Autodesk Inventor part; units mm, degrees
ref_plane "YZ Plane" through (0, 0, 0) normal (1, 0, 0) x (0, 1, 0)
ref_plane "XZ Plane" through (0, 0, 0) normal (0, 1, 0) x (-1, 0, 0)
ref_plane "XY Plane" through (0, 0, 0) normal (0, 0, 1) x (1, 0, 0)
sketch "Esquisse1" plane through (0, 0, 0) normal (0, 1, 0) x (-1, 0, 0)
  line L0 (0, 0) -> (37, 0)
  line L1 (37, 0) -> (37, -31.5)
  line L2 (37, -31.5) -> (0, -31.5)
  line L3 (0, -31.5) -> (0, 0)
  line L4 (34, -28.5) -> (34, -3)
  line L5 (34, -3) -> (3, -3)
  line L6 (3, -3) -> (3, -28.5)
  line L7 (3, -28.5) -> (34, -28.5)
  line L8 (3, -15.75) -> (0, -15.75)
  line L9 (34, -15.75) -> (37, -15.75)
  dimension "d0" = 3
  dimension "d1" = 31
  dimension "d2" = 25.5
extrude "Extrusion1" add sketch "Esquisse1" along normal blind 66 contours L0 L1 L9 L4 L5 L6 L8 L3
sketch "Esquisse2" plane through (-37, 0, 0) normal (0, 0, 1) x (1, 0, 0)
  line L0 (7.5, 22.5) -> (29.5, 22.5) construction
  circle A0 centre (7.5, 22.5) radius 1.65
  circle A1 centre (29.5, 22.5) radius 1.65
  line L1 (34, 0) -> (3, 0) construction
  line L2 (18.5, 0) -> (18.5, 22.5) construction
  point P0 (37, 0)
  dimension "d36" = 4
  dimension "d5" = 3.3
  dimension "d6" = 22.5
  dimension "d7" = 22
extrude "Extrusion2" cut sketch "Esquisse2" against normal through all
sketch "Esquisse3" plane through (-33, 0, 0) normal (0, 0, 1) x (1, 0, 0)
  line L0 (-4, 66) -> (33, 66) construction
  line L1 (-4, 0) -> (33, 0) construction
  circle A0 centre (3.5, 22.5) radius 1.65 construction
  circle A1 centre (25.5, 22.5) radius 1.65 construction
  circle A2 centre (3.5, 22.5) radius 1.65 construction
  circle A3 centre (3.5, 22.5) radius 3.15
  circle A4 centre (25.5, 22.5) radius 3.15
  line L2 (33, 0) -> (33, 66)
  line L3 (-4, 0) -> (-4, 66)
  dimension "d11" = 6.3
extrude "Extrusion3" cut sketch "Esquisse3" against normal blind 1
sketch "Esquisse4" plane through (-33, 0, 0) normal (0, 0, 1) x (1, 0, 0)
  line L0 (-4, 66) -> (33, 66) construction
  line L1 (14.5, 66) -> (14.5, 0) construction
  line L2 (30, 0) -> (-1, 0) construction
  circle A0 centre (14.5, 11) radius 3.5
  circle A1 centre (14.5, 33) radius 3.5
  circle A2 centre (14.5, 55) radius 3.5
  point P0 (33, 0)
  point P1 (0, 56.5)
  point P2 (29, 56.5)
  point P3 (33, 66)
  dimension "d14" = 11
  dimension "d15" = 7
  dimension "d31" = 22
extrude "Extrusion4" cut sketch "Esquisse4" against normal through all
fillet "Congé4" radius 4 2 edges at (0, 33, 0) (-37, 33, 0)
properties part number "part2_top"
Input: part model. Units: mm. Frame: model coordinates. A direction names the side the tool comes from. Round coordinates to 2 decimals unless told otherwise and drop trailing zeros. Write each loop counter-clockwise with the first axis right and the second up, starting at its lowest first coordinate (ties: lowest second). Pieces come first, ordered by that corner, then holes. Notation, with made-up numbers: (-1.5, 54.5) - (23.5, 54.5) arc R23 ccw to (23.5, 85.5) - close; hole circle Ø4 at (-9.5, 27). An arc over 180 degrees is marked (long way). Write item = value, one per line.
(1) Section query D-D on x = -7.5. Output: boundary loops of the cut face in (y, z).
Geometry check:
outline = (0, -3) - (20.85, -3) - (20.85, -1) - (19.35, -1) - (19.35, 0) - (0, 0) - close; (24.15, -3) - (66, -3) - (66, 0) - (25.65, 0) - (25.65, -1) - (24.15, -1) - close
(2) Section query C-C on y = 55. Output: boundary loops of the cut face in (x, z).
Geometry check:
outline = (-37, -15.75) - (-34, -15.75) - (-34, -3) - (-22, -3) - (-22, 0) - (-33, 0) arc R4 ccw to (-37, -4) - close; (-15, -3) - (-3, -3) - (-3, -15.75) - (0, -15.75) - (0, -4) arc R4 ccw to (-4, 0) - (-15, 0) - close
(3) Pull-direction query (Y, two-part tool) for faces 1 (the flat face through (-28, 21, -1)), 2 (the flat face through (-25, 33, 0)); classes: +Y half, -Y half, draft (parallel to the pull), parting line (faces both ways), or undercut.
Geometry check:
face_1 = undercut
face_2 = draft
(4) Material intervals for probe 1 along Y at (x, z) = (-18.5, -2.3); probe 2 along Y at (x, z) = (-29.5, -2.1); probe 3 along X at (y, z) = (3, -12.5), sorted ascending.
Geometry check:
probe_1 = 0 to 7.5, 14.5 to 29.5, 36.5 to 51.5, 58.5 to 66
probe_2 = 0 to 20.85, 24.15 to 66
probe_3 = -37 to -34, -3 to 0
(5) Section query A-A on z = -7. Output: boundary loops of the cut face in (x, y), then the cut area to 3 significant figures.
Geometry check:
outline = (-37, 0) - (-34, 0) - (-34, 66) - (-37, 66) - close; (-3, 0) - (0, 0) - (0, 66) - (-3, 66) - close
area = 396 mm^2
(6) Access query for faces 3 (the cylindrical face through (-9.82, 24.63, -0.49)), 4 (the cylindrical face through (-30.716, 23.615, -1.986)), 5 (the flat face through (-34, 33, -9)). Directions: +Z, -Z, +X, -X, +Y, -Y. A direction counts if a zero-diameter tool reaches every point of the face in a straight line with its end or side. Return the directions, or none.
Geometry check:
face_3 = +Z
face_4 = +Z, -Z
face_5 = -Z, +Y, -Y
(7) Section query B-B on x = -18.5. Output: boundary loops of the cut face in (y, z), then the cut area to 3 significant figures.
Geometry check:
outline = (0, -3) - (7.5, -3) - (7.5, 0) - (0, 0) - close; (14.5, -3) - (29.5, -3) - (29.5, 0) - (14.5, 0) - close; (36.5, -3) - (51.5, -3) - (51.5, 0) - (36.5, 0) - close; (58.5, -3) - (66, -3) - (66, 0) - (58.5, 0) - close
area = 135 mm^2
(8) Contact query for flat-ended pins moving along their axis: pin 1 Ø1.9 at (x, y) = (-30.5, 22) entering from +Z; pin 2 Ø4.5 at (x, y) = (-7.5, 22.5) entering from -Z. Output: stop coordinate, or through.
Geometry check:
pin_1 = -1
pin_2 = -3
